Design review of the part built by this model. Coordinates are the model's own, in mm. A direction names the side the tool comes from. Give positions to 0.01 mm unless a question says otherwise; leave off trailing zeros. Write each loop counter-clockwise with the first axis right and the second up, starting at its lowest first coordinate (ties: lowest second). Pieces come first, ordered by that corner, then holes. Notation, with made-up numbers: M -7.75,5 L 43.25,5 A20 ccw 43.25,10 Z; hole C 10.25,-37.75 d1. An arc over 180 degrees is marked long. Write each question's results on one line, items separated by ' | '. Start each with the question number.
from build123d import *

# Parameters (mm, degrees)
F0_R     = 6.5
F1_DEPTH = 1.4
F2_W     = 15
F2_H     = 1
F3_DEPTH = 2
F4_R     = 0.49999


# Not quite as in the source:
# - a fillet or chamfer is up to 0.001 mm smaller than in the source, because OpenCascade refuses the exact size


with BuildPart() as f1:
    # F0 (on Front) → F1 (new body)
    with BuildSketch(Plane.XZ):
        Polygon((11.5, 20), (-11.5, 20), (-11.5, -20), (-6.5, -20), (-6.5, -25), (6.5, -25), (6.5, -20), (11.5, -20), align=None)
        Circle(F0_R, mode=Mode.SUBTRACT)
    extrude(amount=F1_DEPTH)

    # F2 (on face) → F3 (join)
    with BuildSketch(Plane(origin=(0, 0, 0), x_dir=(-1, 0, 0), z_dir=(0, 1, 0))):
        with Locations((0, 17.9)):
            Rectangle(F2_W, F2_H)
        with Locations((0, -17.9)):
            Rectangle(F2_W, F2_H)
    extrude(amount=F3_DEPTH)

    # F4 (radius 0.5 in the source; OpenCascade refuses exactly that, so slightly less here)
    f4_edges = [f1.edges().sort_by_distance(p)[0] for p in [
        (-6.5, -0.7, -25),
        (6.5, -0.7, -25),
        (0, 0, -25),
        (0, -1.4, -25),
        (6.5, -0.7, -20),
        (6.5, 0, -22.5),
        (6.5, -1.4, -22.5),
        (11.5, -0.7, -20),
        (11.5, -0.7, 20),
        (11.5, 0, 0),
        (11.5, -1.4, 0),
        (-11.5, 0, 0),
        (-6.5, -0.7, -20),
        (-6.5, 0, -22.5),
        (-6.5, -1.4, -22.5),
        (-11.5, -0.7, -20),
        (-9, 0, -20),
        (-9, -1.4, -20),
        (0, 0, 20),
        (0, 2, 17.4),
        (-7.5, 2, 17.9),
        (0, 2, 18.4),
        (7.5, 2, 17.9),
        (-7.5, 2, -17.9),
        (0, 2, -17.4),
        (7.5, 2, -17.9),
        (0, 2, -18.4),
        (9, 0, -20),
        (9, -1.4, -20),
    ]]
    fillet(f4_edges, radius=F4_R)


solid = f1.part
Q1. We need section C-C on z = 0. Write out the cut boundary in (x, y).
Q2. We need section D-D on z = -9.5. Write out the cut boundary in (x, y).
Q3. The part is to be moulded in two halves that separate along X. For faces 6 (the flat face through (0, 1, 17.4)), 7 (the flat face through (7.5, 1, 18)), 8 (the cylindrical face through (-5.158, -0.69, -3.955)), say which applies: pulls with the +X half, pulls with the -X half, needs draft (parallel to the pull), parting line crosses it, or undercut.
Q4. Wall thickness on line 1 along Z through (x, y) = (0, -0.8); line 2 along Z through (x, y) = (5.75, 0.75); line 3 along Y through (x, z) = (-9.5, -14): over which ranges is each line inside the solid? List them lowest first. Write a range as from..to.
Q5. We need section B-B on y = 0.85. Write out the cut boundary in (x, z), and give its area (3 significant figures).
Q6. For pin 1 Ø1 at (x, z) = (6, -10) entering from +Y; pin 2 Ø0.5 at (y, z) = (0.5, 17.5) entering from -X; pin 3 Ø0.5 at (x, y) = (3.5, 0.5) entering from +Z, all flat-tipped, find the tip position at first contact; note any pin that passes through.
Q7. For faces 1 (the flat face through (0, 1, -18.4)), 2 (the flat face through (0, 1, -17.4)), 3 (the flat face through (-7.5, 1, 18)), 4 (the flat face through (0, 1, 18.4)), 5 (the flat face through (7.5, 1, -18)), list the 3-axis set-ups (+Z, -Z, +X, -X, +Y, -Y) from which the entire face can be reached by the end or side of a thin tool; tool diameter is ignored.
Answer sheet:
1) outline: M -11.5,-1.4 L -6.5,-1.4 L -6.5,0 L -11,0 A0.5 ccw -11.5,-0.5 Z; M 6.5,-1.4 L 11,-1.4 A0.5 ccw 11.5,-0.9 L 11.5,-0.5 A0.5 ccw 11,0 L 6.5,0 Z
2) outline: M -11.5,-1.4 L 11,-1.4 A0.5 ccw 11.5,-0.9 L 11.5,-0.5 A0.5 ccw 11,0 L -11,0 A0.5 ccw -11.5,-0.5 Z
3) face 6: needs draft | face 7: pulls with the +X half | face 8: undercut
4) line 1: -25..-6.5, 6.5..20 | line 2: -18.4..-17.4, 17.4..18.4 | line 3: -1.4..0
5) outline: M -7.5,-18.4 L 7.5,-18.4 L 7.5,-17.4 L -7.5,-17.4 Z; M -7.5,17.4 L 7.5,17.4 L 7.5,18.4 L -7.5,18.4 Z | area: 30.0 mm^2
6) pin 1: y = 0 | pin 2: x = -7.5 | pin 3: z = 18.4
7) face 1: -Z, +X, -X, +Y | face 2: +X, -X, +Y | face 3: +Z, -Z, -X, +Y | face 4: +Z, +X, -X, +Y | face 5: +Z, -Z, +X, +Y
